Here's how the part is built. I have some questions about the finished solid (model axes, mm). A direction names the side the tool comes from. Round coordinates to 2 decimals unless told otherwise and drop trailing zeros. Write each loop counter-clockwise with the first axis right and the second up, starting at its lowest first coordinate (ties: lowest second). Pieces come first, ordered by that corner, then holes. Notation, with made-up numbers: M -15.75,5.5 L 17.25,5.5 A21 ccw 17.25,22.5 Z; hole C -36,10.25 d2. An arc over 180 degrees is marked long. Use a Markdown table: item, result. Add a question column.
```python
from build123d import *

# Parameters (mm, degrees)
SKETCH1_R              = 1.75
BOSS_EXTRUDE1_DEPTH    = 2
SKETCH2_W              = 7
SKETCH2_H              = 16
BOSS_EXTRUDE2_DEPTH    = 14
CUT_EXTRUDE1_DEPTH     = 50.658836072
SKETCH5_W              = 15
SKETCH5_H              = 2.5
BOSS_EXTRUDE3_DEPTH    = 6
CUT_EXTRUDE2_DEPTH     = 44.33589736
FILLET2_R              = 2
SKETCH7_R              = 3
CUT_EXTRUDE3_DEPTH     = 44.33589736
SKETCH8_W              = 26
SKETCH8_H              = 18
SKETCH8_R              = 1.75
PINOUT_BD_HOLDER_DEPTH = 2
WEIGH_REDUCER_DEPTH    = 53.318734694
FILLET3_R              = 4
FILLET4_R              = 2
FILLET5_DEPTH          = 2
FILLET5_START          = -7.5
FILLET5_2_DEPTH        = 15
FILLET5_START_2        = -1
FILLET5_3_DEPTH        = 4


with BuildPart() as part:
    # Sketch1 → Boss-Extrude1 (new body)
    with BuildSketch(Plane(origin=(0, 0, 0), x_dir=(1, 0, 0), z_dir=(0, 1, 0))):
        with BuildLine():
            Line((-25, 29), (25, 29))
            ThreePointArc((25, 29), (27.828427125, 27.828427125), (29, 25))
            Line((29, 25), (29, -25))
            ThreePointArc((29, -25), (27.828427125, -27.828427125), (25, -29))
            Line((25, -29), (-25, -29))
            ThreePointArc((-25, -29), (-27.828427125, -27.828427125), (-29, -25))
            Line((-29, -25), (-29, 25))
            ThreePointArc((-29, 25), (-27.828427125, 27.828427125), (-25, 29))
        make_face()
        with Locations(Location((23.75, 23.75, 0), (0, 0, 270))):
            Circle(SKETCH1_R, mode=Mode.SUBTRACT)
        with Locations(Location((23.75, -23.75, 0), (0, 0, 270))):
            Circle(SKETCH1_R, mode=Mode.SUBTRACT)
        with Locations(Location((-23.75, -23.75, 0), (0, 0, 270))):
            Circle(SKETCH1_R, mode=Mode.SUBTRACT)
        with Locations(Location((-23.75, 23.75, 0), (0, 0, 270))):
            Circle(SKETCH1_R, mode=Mode.SUBTRACT)
        with BuildLine():
            Line((-12, 14), (12, 14))
            ThreePointArc((12, 14), (13.414213562, 13.414213562), (14, 12))
            Line((14, 12), (14, -12))
            ThreePointArc((14, -12), (13.414213562, -13.414213562), (12, -14))
            Line((12, -14), (-12, -14))
            ThreePointArc((-12, -14), (-13.414213562, -13.414213562), (-14, -12))
            Line((-14, -12), (-14, 12))
            ThreePointArc((-14, 12), (-13.414213562, 13.414213562), (-12, 14))
        make_face(mode=Mode.SUBTRACT)
    extrude(amount=BOSS_EXTRUDE1_DEPTH)

    # Sketch2 → Boss-Extrude2 (add)
    with BuildSketch(Plane(origin=(0, 2, 0), x_dir=(1, 0, 0), z_dir=(0, 1, 0))):
        with Locations((-22, 0)):
            Rectangle(SKETCH2_W, SKETCH2_H)
        with Locations((22, 0)):
            Rectangle(SKETCH2_W, SKETCH2_H)
    extrude(amount=BOSS_EXTRUDE2_DEPTH)

    # Sketch4 → Cut-Extrude1 (cut, through all)
    with BuildSketch(Plane.XY.offset(8)):
        Polygon((-18.5, 16), (-22.5, 16), (-22.5, 8), (-18.5, 2), align=None)
        Polygon((18.5, 2), (18.5, 16), (22.5, 16), (22.5, 8), align=None)
    extrude(amount=-CUT_EXTRUDE1_DEPTH, mode=Mode.SUBTRACT)

    # Sketch5 → Boss-Extrude3 (add)
    with BuildSketch(Plane(origin=(0, 2, 0), x_dir=(1, 0, 0), z_dir=(0, 1, 0))):
        with Locations((0, 21.25)):
            Rectangle(SKETCH5_W, SKETCH5_H)
        with Locations((0, -21.25)):
            Rectangle(SKETCH5_W, SKETCH5_H)
    extrude(amount=BOSS_EXTRUDE3_DEPTH)

    # Sketch6 → Cut-Extrude2 (cut, through all)
    with BuildSketch(Plane(origin=(0, 2, 0), x_dir=(1, 0, 0), z_dir=(0, 1, 0))):
        Polygon((-25.5, 8), (-25.5, 17), (-29, 22), (-29, -22), (-25.5, -17), (-25.5, -8), align=None)
        Polygon((-15.45, -22.5), (-7.5, -22.5), (7.5, -22.5), (15.45, -22.5), (20, -29), (-20, -29), align=None)
        Polygon((29, 22), (29, -22), (25.5, -17), (25.5, -8), (25.5, 8), (25.5, 17), align=None)
        Polygon((-7.5, 22.5), (7.5, 22.5), (15.45, 22.5), (20, 29), (-20, 29), (-15.45, 22.5), align=None)
    extrude(amount=-CUT_EXTRUDE2_DEPTH, mode=Mode.SUBTRACT)

    # Fillet2
    fillet2_edges = [part.edges().sort_by_distance(p)[0] for p in [
        (-25.5, 1, -17),
        (-25.5, 1, 17),
        (-29, 1, 22),
        (-29, 1, -22),
        (-20, 1, 29),
        (-15.45, 1, 22.5),
        (15.45, 1, 22.5),
        (20, 1, 29),
        (25.5, 1, -17),
        (29, 1, -22),
        (29, 1, 22),
        (25.5, 1, 17),
        (-15.45, 1, -22.5),
        (-20, 1, -29),
        (20, 1, -29),
        (15.45, 1, -22.5),
    ]]
    fillet(fillet2_edges, radius=FILLET2_R)

    # Sketch7 → Cut-Extrude3 (cut, through all)
    with BuildSketch(Plane(origin=(0, 2, 0), x_dir=(1, 0, 0), z_dir=(0, 1, 0))):
        with Locations(Location((19.5, 16, 0), (0, 0, 270))):
            Circle(SKETCH7_R)
        with Locations(Location((19.5, -16, 0), (0, 0, 90))):
            Circle(SKETCH7_R)
        with Locations(Location((-19.5, -16, 0), (0, 0, 270))):
            Circle(SKETCH7_R)
        with Locations(Location((-19.5, 16, 0), (0, 0, 90))):
            Circle(SKETCH7_R)
    extrude(amount=-CUT_EXTRUDE3_DEPTH, mode=Mode.SUBTRACT)

    # Sketch8 → pinout_bd_holder (add)
    with BuildSketch(Plane(origin=(0, 2, 0), x_dir=(1, 0, 0), z_dir=(0, 1, 0))):
        with Locations((0, 31.5)):
            Rectangle(SKETCH8_W, SKETCH8_H)
        with Locations(Location((-10, 37, 0), (0, 0, 270))):
            Circle(SKETCH8_R, mode=Mode.SUBTRACT)
        with Locations(Location((10, 37, 0), (0, 0, 90))):
            Circle(SKETCH8_R, mode=Mode.SUBTRACT)
    extrude(amount=-PINOUT_BD_HOLDER_DEPTH)

    # Sketch9 → Weigh-Reducer (cut, through all)
    with BuildSketch(Plane.XZ):
        with BuildLine():
            Line((-7.5, -24), (7.5, -24))
            ThreePointArc((7.5, -24), (8.560660172, -24.439339828), (9, -25.5))
            Line((9, -25.5), (9, -32))
            ThreePointArc((9, -32), (8.560660172, -33.060660172), (7.5, -33.5))
            Line((7.5, -33.5), (6.5, -33.5))
            ThreePointArc((6.5, -33.5), (5.439339828, -33.939339828), (5, -35))
            Line((5, -35), (5, -36))
            ThreePointArc((5, -36), (4.560660172, -37.060660172), (3.5, -37.5))
            Line((3.5, -37.5), (-3.5, -37.5))
            ThreePointArc((-3.5, -37.5), (-4.560660172, -37.060660172), (-5, -36))
            Line((-5, -36), (-5, -35))
            ThreePointArc((-5, -35), (-5.439339828, -33.939339828), (-6.5, -33.5))
            Line((-6.5, -33.5), (-7.5, -33.5))
            ThreePointArc((-7.5, -33.5), (-8.560660172, -33.060660172), (-9, -32))
            Line((-9, -32), (-9, -25.5))
            ThreePointArc((-9, -25.5), (-8.560660172, -24.439339828), (-7.5, -24))
        make_face()
    extrude(amount=-WEIGH_REDUCER_DEPTH, mode=Mode.SUBTRACT)

    # Fillet3
    fillet3_edges = [part.edges().sort_by_distance(p)[0] for p in [
        (22.5, 8, 0),
        (-18.5, 2, 0),
        (18.5, 2, 0),
        (-22.5, 8, 0),
    ]]
    fillet(fillet3_edges, radius=FILLET3_R)

    # Fillet4
    fillet4_edges = [part.edges().sort_by_distance(p)[0] for p in [
        (0, 2, -20),
        (0, 2, 20),
    ]]
    fillet(fillet4_edges, radius=FILLET4_R)

    # Fillet5: read off the stored shape, not the designer's step
    # Fillet5 outline → Fillet5 (add)
    with BuildSketch(Plane(origin=(0, 0, 0), x_dir=(1, 0, 0), z_dir=(0, 1, 0))):
        with BuildLine():
            Line((-13, 22.5), (-13, 24.410589217))
            ThreePointArc((-13, 24.410589217), (-13.390245011, 23.223707219), (-14.408688877, 22.5))
            Line((-14.408688877, 22.5), (-13, 22.5))
        make_face()
        with BuildLine():
            ThreePointArc((14.408688877, 22.5), (13.390245011, 23.223707219), (13, 24.410589217))
            Line((13, 24.410589217), (13, 22.5))
            Line((13, 22.5), (14.408688877, 22.5))
        make_face()
    extrude(amount=FILLET5_DEPTH)

    # Fillet5 2 outline → Fillet5 2 (add)
    with BuildSketch(Plane.YZ.offset(FILLET5_START)):
        with BuildLine():
            ThreePointArc((2, -24), (2.711746802, -22.91886117), (3.936491673, -22.5))
            Line((3.936491673, -22.5), (2, -22.5))
            Line((2, -22.5), (2, -24))
        make_face()
    extrude(amount=FILLET5_2_DEPTH)

    # Fillet5 3 outline → Fillet5 3 (cut)
    with BuildSketch(Plane(origin=(0, 0, 0), x_dir=(1, 0, 0), z_dir=(0, 1, 0)).offset(FILLET5_START_2)):
        with BuildLine():
            ThreePointArc((-13, 38.5), (-12.414213562, 39.914213562), (-11, 40.5))
            Line((-11, 40.5), (-13, 40.5))
            Line((-13, 40.5), (-13, 38.5))
        make_face()
        with BuildLine():
            ThreePointArc((11, 40.5), (12.414213562, 39.914213562), (13, 38.5))
            Line((13, 38.5), (13, 40.5))
            Line((13, 40.5), (11, 40.5))
        make_face()
    extrude(amount=FILLET5_3_DEPTH, mode=Mode.SUBTRACT)


solid = part.part
```
Item 1: If we mould it in two halves opening along X, with no side actions, what happens to faces 5 (the face through (-27.859, 0.986, -27.797)), 6 (the face through (-23, 7, -8)), 7 (the face through (14, 1, 0))? For each: +X half, -X half, draft (parallel to the pull), parting line (faces both ways), or undercut.
Item 2: I need wall thicknesses on probe 1 along X at (y, z) = (1.4, -16); probe 2 along Y at (x, z) = (11.5, -19); probe 3 along X at (y, z) = (12.75, 4). Which ranges of each line are inside material? Lowest first, please. Write a range as from..to.
Item 3: Imagine slicing it at A-A on z = -31. List the corners of the cut face in (x, y) for me, plus the area to 3 significant figures.
Item 4: Imagine slicing it at D-D on z = -3. List the corners of the cut face in (x, y) for me, plus the area to 3 significant figures.
Item 5: For pin 1 Ø0.6 at (y, z) = (1.5, 3) entering from +X; pin 2 Ø0.6 at (x, y) = (-0.5, 0.5) entering from +Z; pin 3 Ø2 at (y, z) = (11.5, -1) entering from -X, each with a flat end and sliding along its axis, tell me the tip position at first contact or that it passes through.
Item 6: Imagine slicing it at C-C on y = 12. List the corners of the cut face in (x, z) for me, plus the area to 3 significant figures.
Item 7: Imagine slicing it at B-B on x = -2.5. List the corners of the cut face in (y, z) for me.
Item 8: On a 3-axis mill with a long thin cutter (end or side, diameter ignored), from which of +Z, -Z, +X, -X, +Y, -Y can I reach the whole of each face in a straight line? I mean faces 1 (the face through (8.57, 0.99, -33.05)), 2 (the face through (27.23, 1.01, -19.47)), 3 (the face through (23, 1, -29)), 4 (the face through (13.4, 0.99, -23.21)). Say none if no direction works.
The answers:
| question | item | result |
|---|---|---|
| 1 | face 5 | -X half |
| 1 | face 6 | draft |
| 1 | face 7 | undercut |
| 2 | probe 1 | -25.5..-22.5, -16.5..16.5, 22.5..25.5 |
| 2 | probe 2 | 0..2 |
| 2 | probe 3 | -25.5..-22.5, 22.5..25.5 |
| 3 | outline | M -13,0 L -9,0 L -9,2 L -13,2 Z; M 9,0 L 13,0 L 13,2 L 9,2 Z |
| 3 | area | 16.0 mm² |
| 4 | outline | M -25.5,0 L -14,0 L -14,2 L -16.36,2 A4 cw -19.69,3.78 L -21.83,6.99 A4 cw -22.5,9.21 L -22.5,16 L -25.5,16 Z; M 14,0 L 25.5,0 L 25.5,16 L 22.5,16 L 22.5,9.21 A4 cw 21.83,6.99 L 19.69,3.78 A4 cw 16.36,2 L 14,2 Z |
| 4 | area | 156 mm² |
| 5 | pin 1 | x = 25.5 |
| 5 | pin 2 | z = 22.5 |
| 5 | pin 3 | x = -25.5 |
| 6 | outline | M -25.5,-8 L -22.5,-8 L -22.5,8 L -25.5,8 Z; M 22.5,-8 L 25.5,-8 L 25.5,8 L 22.5,8 Z |
| 6 | area | 96.0 mm² |
| 7 | outline | M 0,-40.5 L 2,-40.5 L 2,-37.5 L 0,-37.5 Z; M 0,-24 L 2,-24 A2 cw 3.94,-22.5 L 8,-22.5 L 8,-20 L 4,-20 A2 cw 2,-18 L 2,-14 L 0,-14 Z; M 0,14 L 2,14 L 2,18 A2 cw 4,20 L 8,20 L 8,22.5 L 0,22.5 Z |
| 8 | face 1 | +Y, -Y |
| 8 | face 2 | +X, +Y, -Y |
| 8 | face 3 | -Z, +X, +Y, -Y |
| 8 | face 4 | -Z, +Y, -Y |
